from build123d import *

# Parameters (mm, degrees)
SKETCH3_W = 0.254
SKETCH3_H = 0.508


with BuildPart() as part:
    # Sketch1 → Revolve1 (revolve)
    with BuildSketch(Plane.XY):
        Polygon((0, 0), (0, 1.5875), (39.243, 1.5875), (39.243, 4.03225), (51.0794, 4.03225), (51.0794, 0), align=None)
    revolve(axis=Axis((51.0794, 0, 0), (-1, 0, 0)))

    # Sketch2 → Revolve2 (revolve)
    with BuildSketch(Plane.XY):
        Polygon((-9.652, 0), (-9.652, 1.20904), (-9.27354, 1.5875), (0, 1.5875), (0, 0), align=None)
    revolve(axis=Axis((0, 0, 0), (-1, 0, 0)))

    # Sketch3 → Cut-Revolve1 (revolve, cut)
    with BuildSketch(Plane.XY):
        with Locations((-0.127, 1.5875)):
            Rectangle(SKETCH3_W, SKETCH3_H)
    revolve(axis=Axis((0, 0, 0), (-1, 0, 0)), mode=Mode.SUBTRACT)


solid = part.part
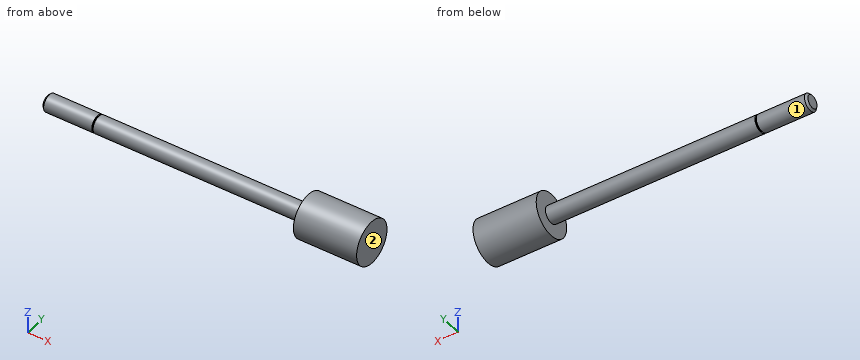
For this review, take the finished solid that the model builds, in its own axes (mm). Face numbers are marked on the shaded views. A direction names the side the tool comes from. Give positions to 0.01 mm unless a question says otherwise; leave off trailing zeros. Loops run counter-clockwise (first coordinate to the right, second up) from the corner with the lowest first, then second, coordinate; pieces in that order, holes last. Notation, with made-up numbers: (18.25, 69.25) -> (29.25, 69.25) arc R8 cw to (29.25, 83.25) -> close; hole circle Ø4 at (33, 31). An arc over 180 degrees is marked (long way). One line per question, with ' | ' between items.
1) For the marked faces 1 and 2, list the 3-axis set-ups (+Z, -Z, +X, -X, +Y, -Y) from which the entire face can be reached by the end or side of a thin tool; tool diameter is ignored.
Resolved:
face 1: -X | face 2: +Z, -Z, +X, +Y, -Y
2) We need section A-A (z = 0). Write out the cut boundary in (x, y).
Resolved:
outline: (-9.65, -1.21) -> (-9.27, -1.59) -> (-0.25, -1.59) -> (-0.25, -1.33) -> (0, -1.33) -> (0, -1.59) -> (39.24, -1.59) -> (39.24, -4.03) -> (51.08, -4.03) -> (51.08, 4.03) -> (39.24, 4.03) -> (39.24, 1.59) -> (0, 1.59) -> (0, 1.33) -> (-0.25, 1.33) -> (-0.25, 1.59) -> (-9.27, 1.59) -> (-9.65, 1.21) -> close
3) To check wall thickness, follow probe 1 along X at (y, z) = (0.5, -1.75); probe 2 along Z at (x, y) = (22, 0.75); probe 3 along Z at (x, y) = (6, 0.5). State the ranges of each line that lie inside material, in increasing order.
Resolved:
probe 1: x = 39.24 to 51.08 | probe 2: z = -1.4 to 1.4 | probe 3: z = -1.51 to 1.51
4) We need section C-C (x = 29.5). Write out the cut boundary in (y, z) (1 decimal), plus the area to 3 significant figures.
Resolved:
outline: circle Ø3.2 at (0, 0) | area: 7.92 mm2
5) We need section D-D (z = 2.5). Write out the cut boundary in (x, y).
Resolved:
outline: (39.24, -3.16) -> (51.08, -3.16) -> (51.08, 3.16) -> (39.24, 3.16) -> close
6) Insertion check: pin 1 Ø2 at (x, y) = (14.5, 0.5) entering from -Z; pin 2 Ø2 at (x, y) = (38.5, -1) entering from +Z. Each pin has a flat end and moves straight along its axis. Give the tip position at first contact, or say it passes through.
Resolved:
pin 1: stops at z = -1.59 | pin 2: stops at z = 4.02
